```python
from build123d import *

# Parameters (mm, degrees)
F0_W     = 25.6
F0_H     = 57.6
F0_W_2   = 21.6
F0_H_2   = 53.6
F1_DEPTH = 1
F0_W_3   = 11
F0_H_3   = 2
F2_DEPTH = 3
F3_DEPTH = 5
F4_R     = 2
F5_R     = 0.2


with BuildPart() as f1:
    # F0 (on Top) → F1 (new body)
    with BuildSketch(Plane.XY):
        with Locations((0, -1.2393394568)):
            Rectangle(F0_W, F0_H)
        with Locations((0, -1.2393394568)):
            Rectangle(F0_W_2, F0_H_2, mode=Mode.SUBTRACT)
    extrude(amount=F1_DEPTH)

    # F0 (on Top) → F2 (join)
    with BuildSketch(Plane.XY):
        with Locations((0, -1.2393394568)):
            Rectangle(F0_W_2, F0_H_2)
        with Locations((0, -7.1393394568)):
            Rectangle(F0_W_3, F0_H_3, mode=Mode.SUBTRACT)
    extrude(amount=F2_DEPTH)

    # F0 (on Top) → F3 (join)
    with BuildSketch(Plane.XY):
        with Locations((0, -7.1393394568)):
            Rectangle(F0_W_3, F0_H_3)
    extrude(amount=F3_DEPTH)

    # F4
    f4_edges = [f1.edges().sort_by_distance(p)[0] for p in [
        (-12.8, -30.039339, 0.5),
        (12.8, -30.039339, 0.5),
        (12.8, 27.560661, 0.5),
        (-12.8, 27.560661, 0.5),
    ]]
    fillet(f4_edges, radius=F4_R)

    # F5
    f5_edges = [f1.edges().sort_by_distance(p)[0] for p in [
        (12.8, -1.239339, 1),
        (0, -28.039339, 3),
        (10.8, -1.239339, 3),
        (0, 25.560661, 3),
        (-10.8, -1.239339, 3),
        (-5.5, -7.139339, 3),
        (0, -6.139339, 3),
        (5.5, -7.139339, 3),
        (0, -8.139339, 3),
        (10.8, 25.560661, 2),
        (-10.8, 25.560661, 2),
        (-10.8, -28.039339, 2),
        (10.8, -28.039339, 2),
        (0, -6.139339, 5),
        (-5.5, -7.139339, 5),
        (0, -8.139339, 5),
        (5.5, -7.139339, 5),
        (5.5, -8.139339, 4),
        (-5.5, -8.139339, 4),
        (5.5, -6.139339, 4),
        (-5.5, -6.139339, 4),
    ]]
    fillet(f5_edges, radius=F5_R)


solid = f1.part
```
Design review of the part built by this model. Coordinates are the model's own, in mm. A direction names the side the tool comes from. Give positions to 0.01 mm unless a question says otherwise; leave off trailing zeros. Write each loop counter-clockwise with the first axis right and the second up, starting at its lowest first coordinate (ties: lowest second). Pieces come first, ordered by that corner, then holes. Notation, with made-up numbers: (-20, -21.5) - (12, -21.5) arc R24 ccw to (12, 10.5) - close; hole circle Ø10 at (-6.75, 9.25). An arc over 180 degrees is marked (long way). Return JSON: item names as keys, results as strings. Group by question number.
(1) We need section B-B, the plane z = 1.8. Give the boundary of the cut face in (x, y).
(2) We need section A-A, the plane y = -20.5. Give the boundary of the cut face in (x, z), then the cut area to 3 significant figures.
(3) We need section D-D, the plane x = 3. Give the boundary of the cut face in (y, z), then the cut area to 3 significant figures.
(4) Insertion check: pin 1 (6.5 mm diameter, centred on x = -3.5, y = -13.5, fed in from +Z); pin 2 (0.5 mm diameter, centred on y = -2.5, z = 1.5, fed in from -X); pin 3 (1.3 mm diameter, centred on x = 1.5, z = 4, fed in from +Y). Each pin has a flat end and moves straight along its axis. Give the tip position at first contact, or say it passes through.
(5) Machinability: for faces 1 (the flat face through (0, -6.139, 4)), 2 (the flat face through (0, -28.039, 2)), 3 (the flat face through (10.8, -2, 2)), 4 (the flat face through (-10.8, -2, 2)), which of the approach directions +Z, -Z, +X, -X, +Y, -Y give a long, thin tool a straight path to every point of the face, cutting with its end or side? Answer none if there is none.
(6) To check wall thickness, follow probe 1 along Z at (x, y) = (-9.75, -23); probe 2 along Y at (x, z) = (-0.75, 4.35); probe 3 along Y at (x, z) = (-2.25, 1.95). State the ranges of each line that lie inside material, in increasing order.
(7) We need section C-C, the plane x = 9. Give the boundary of the cut face in (y, z).
Reported:
{
 "1": {"outline": "(-10.8, -27.84) arc R0.2 ccw to (-10.6, -28.04) - (10.6, -28.04) arc R0.2 ccw to (10.8, -27.84) - (10.8, 25.36) arc R0.2 ccw to (10.6, 25.56) - (-10.6, 25.56) arc R0.2 ccw to (-10.8, 25.36) - close"},
 "2": {"outline": "(-12.8, 0) - (12.8, 0) - (12.8, 0.8) arc R0.2 ccw to (12.6, 1) - (10.8, 1) - (10.8, 2.8) arc R0.2 ccw to (10.6, 3) - (-10.6, 3) arc R0.2 ccw to (-10.8, 2.8) - (-10.8, 1) - (-12.6, 1) arc R0.2 ccw to (-12.8, 0.8) - close", "area": "68.8 mm2"},
 "3": {"outline": "(-30.04, 0) - (27.56, 0) - (27.56, 0.8) arc R0.2 ccw to (27.36, 1) - (25.56, 1) - (25.56, 2.8) arc R0.2 ccw to (25.36, 3) - (-5.94, 3) arc R0.2 cw to (-6.14, 3.2) - (-6.14, 4.8) arc R0.2 ccw to (-6.34, 5) - (-7.94, 5) arc R0.2 ccw to (-8.14, 4.8) - (-8.14, 3.2) arc R0.2 cw to (-8.34, 3) - (-27.84, 3) arc R0.2 ccw to (-28.04, 2.8) - (-28.04, 1) - (-29.84, 1) arc R0.2 ccw to (-30.04, 0.8) - close", "area": "169 mm2"},
 "4": {"pin 1": "stops at z = 3", "pin 2": "stops at x = -10.8", "pin 3": "stops at y = -6.14"},
 "5": {"face 1": "+Z, +X, -X, +Y", "face 2": "+Z, +X, -X, -Y", "face 3": "+Z, +X, +Y, -Y", "face 4": "+Z, -X, +Y, -Y"},
 "6": {"probe 1": "z = 0 to 3", "probe 2": "y = -8.14 to -6.14", "probe 3": "y = -28.04 to 25.56"},
 "7": {"outline": "(-30.04, 0) - (27.56, 0) - (27.56, 0.8) arc R0.2 ccw to (27.36, 1) - (25.56, 1) - (25.56, 2.8) arc R0.2 ccw to (25.36, 3) - (-27.84, 3) arc R0.2 ccw to (-28.04, 2.8) - (-28.04, 1) - (-29.84, 1) arc R0.2 ccw to (-30.04, 0.8) - close"}
}
